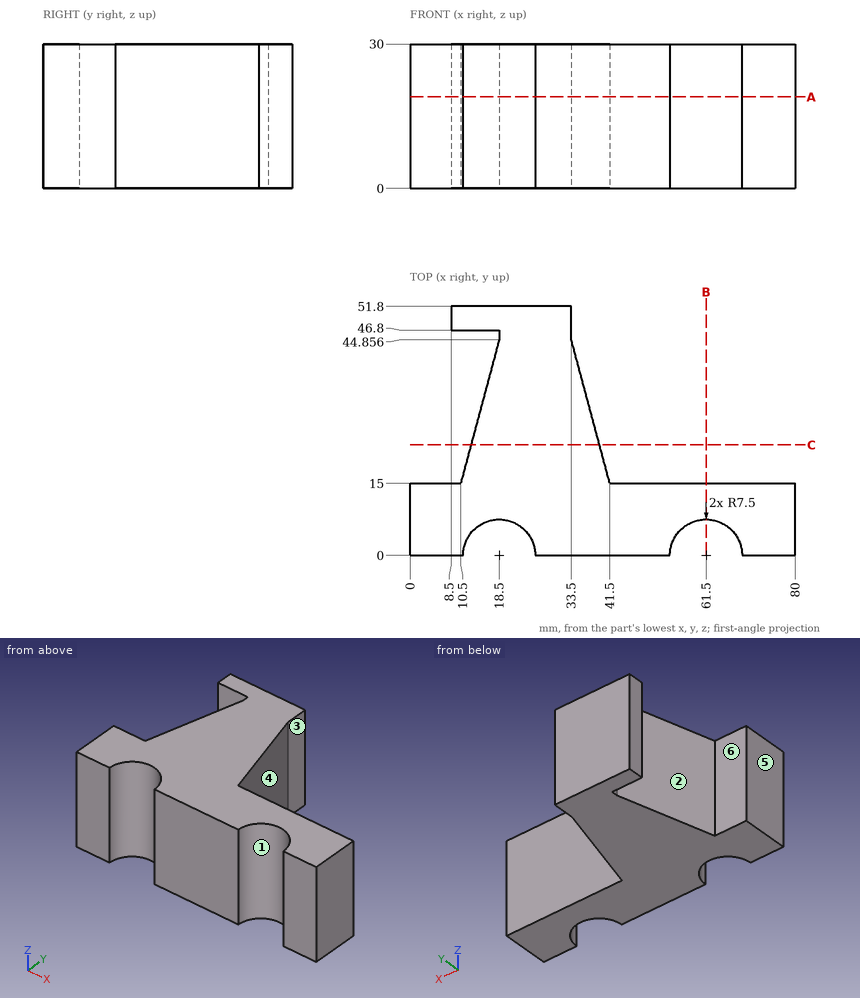
Could you check a few things on this drawing? It's one solid part, dimensions in mm from its lowest x, y, z. A direction names the side the tool comes from. Coordinates: 2 decimals unless noted, no trailing zeros. Write each loop counter-clockwise with the first axis right and the second up, starting at its lowest first coordinate (ties: lowest second). Pieces come first, ordered by that corner, then holes. Notation, with made-up numbers: (-7, -33) - (18, -33) arc R12 cw to (18, -10) - close; hole circle Ø3 at (13.5, 89.5). An arc over 180 degrees is marked (long way). Return JSON: item names as keys, results as strings. Group by question number.
Item 1: We'd pull the mould along Y, two halves only. Please class the marked faces 4, 5 and 6: pulls with the +Y half, pulls with the -Y half, needs draft (parallel to the pull), parting line crosses it, or undercut.
Item 2: I'm going to push flat-ended pins straight in: pin 1 Ø5.5 at (y, z) = (49, 15) entering from -X; pin 2 Ø1 at (y, z) = (46, 14) entering from -X; pin 3 Ø10 at (x, y) = (46, 18.5) entering from +Z; pin 4 Ø4 at (y, z) = (18.5, 9.5) entering from +X. Where does each tip first touch, or does it pass through?
Item 3: Please list where these lines run through material, in increasing order: probe 1 along Y at (x, z) = (48.5, 18); probe 2 along X at (y, z) = (49, 22.5); probe 3 along X at (y, z) = (6.5, 17.5) (1 decimal).
Item 4: If we section it at A-A (z = 19): Write out the boundary of the cut face in (x, y), then the cut area to 3 significant figures.
Item 5: If we section it at B-B (x = 61.5): Write out the boundary of the cut face in (y, z), then the cut area to 3 significant figures.
Item 6: Which directions (+Z, -Z, +X, -X, +Y, -Y) give clear straight access to the entire face, cutting with the end or side of a thin tool? Please do the marked faces 1, 2 and 3.
Item 7: If we section it at C-C (y = 23): Write out the boundary of the cut face in (x, z), then the cut area to 3 significant figures.
Return value:
{
 "1": {"face 4": "pulls with the +Y half", "face 5": "needs draft", "face 6": "undercut"},
 "2": {"pin 1": "stops at x = 8.5", "pin 2": "stops at x = 18.5", "pin 3": "stops at z = 30", "pin 4": "stops at x = 41.1"},
 "3": {"probe 1": "y = 0 to 15", "probe 2": "x = 8.5 to 33.5", "probe 3": "x = 0 to 14.8, 22.2 to 57.8, 65.2 to 80"},
 "4": {"outline": "(0, 0) - (11, 0) arc R7.5 cw to (26, 0) - (54, 0) arc R7.5 cw to (69, 0) - (80, 0) - (80, 15) - (41.5, 15) - (33.5, 44.86) - (33.5, 51.8) - (8.5, 51.8) - (8.5, 46.8) - (18.5, 46.8) - (18.5, 44.86) - (10.5, 15) - (0, 15) - close", "area": "1,860 mm^2"},
 "5": {"outline": "(7.5, 0) - (15, 0) - (15, 30) - (7.5, 30) - close", "area": "225 mm^2"},
 "6": {"face 1": "+Z, -Z, -Y", "face 2": "+Z, -Z, -X", "face 3": "+Z, -Z, +X, +Y"},
 "7": {"outline": "(12.64, 0) - (39.36, 0) - (39.36, 30) - (12.64, 30) - close", "area": "801 mm^2"}
}
